Autodesk Inventor part; units mm, degrees
ref_plane "YZ Plane" through (0, 0, 0) normal (1, 0, 0) x (0, 1, 0)
ref_plane "XZ Plane" through (0, 0, 0) normal (0, 1, 0) x (-1, 0, 0)
ref_plane "XY Plane" through (0, 0, 0) normal (0, 0, 1) x (1, 0, 0)
sketch "Boceto1" plane through (0, 0, 0) normal (0, 1, 0) x (-1, 0, 0)
  circle A0 centre (0, 0) radius 1.55
  line L0 (0, 0) -> (0, -1.55)
  line L1 (0, -19.075) -> (0, -14.075)
  line L2 (0, 19.075) -> (0, 16.575)
  arc A1 (2.4369, 17.1331) -> (-2.4369, 17.1331) centre (0, 16.575) ccw
  line L3 (0, -19.075) -> (0, -16.575)
  arc A2 (-2.4369, -17.1331) -> (2.4369, -17.1331) centre (0, -16.575) ccw
  line L4 (-2.4369, 17.1331) -> (-6.0436, 1.384)
  line L5 (2.4369, 17.1331) -> (6.0436, 1.384)
  line L6 (2.4369, -17.1331) -> (6.0436, -1.384)
  line L7 (-2.4369, -17.1331) -> (-6.0436, -1.384)
  arc A3 (-6.0436, 1.384) -> (-6.0436, -1.384) centre (0, 0) ccw
  arc A4 (6.0436, -1.384) -> (6.0436, 1.384) centre (0, 0) ccw
  dimension "d0" = 3.1
  dimension "d2" = 19.075
  dimension "d3" = 38.15
  dimension "d4" = 2.5
  dimension "d5" = 2.5
extrude "Extrusión1" add sketch "Boceto1" along normal blind 2.3
sketch "Boceto2" plane through (0, 2.3, 0) normal (0, 1, 0) x (1, 0, 0)
  circle A0 centre (0, 0) radius 1.55
  circle A1 centre (0, 0) radius 4.35
  circle A2 centre (0, 0) radius 2.7
  dimension "d8" = 8.7
  dimension "d9" = 5.4
extrude "Extrusión2" add sketch "Boceto2" along normal blind 3.3 contours A1
sketch "Boceto3" plane through (0, 0, 0) normal (0, -1, 0) x (1, 0, 0)
  circle A0 centre (0, 0) radius 1.55
  line L0 (0, -1.55) -> (0, 1.55)
properties part number "Brazo"
CAD build for the part. Positions are in the model's coordinates, mm. Coordinates: 2 decimals unless noted, no trailing zeros. Write each loop counter-clockwise with the first axis right and the second up, starting at its lowest first coordinate (ties: lowest second). Pieces come first, ordered by that corner, then holes.
(1) Flat gauge pins, fed straight in: pin 1 (6 mm diameter, centred on x = 0, z = 2.5, fed in from +Y); pin 2 (2.5 mm diameter, centred on x = 0, z = -0.5, fed in from +Y); pin 3 (2 mm diameter, centred on x = 3, y = 3.5, fed in from +Z). Where does each tip first touch, or does it go through?
(2) Cut at B-B, the plane z = 0. List the corners of the cut face in (x, y), and give its area (3 significant figures).
(3) Two-plate mould, pull along X, no slides. Class faces 1 (the face through (0, 2.3, -2)), 2 (the face through (-0.943, 3.927, -4.247)), 3 (the face through (-0.585, 3.927, -2.636)), 4 (the face through (0, 2.3, 5)): +X half, -X half, draft (parallel to the pull), parting line (faces both ways), or undercut.
(4) Cut at C-C, the plane y = 5.2. List the corners of the cut face in (x, z).
(5) Cut at A-A, the plane x = 0. List the corners of the cut face in (y, z) (3 decimals).
(6) Cut at D-D, the plane x = 4. List the corners of the cut face in (y, z).
(7) Drill centre lines: probe 1 along X at (y, z) = (4.6, 0); probe 2 along Z at (x, y) = (0, 1.3) (3 decimals). Where is each one in solid material? Low to high.
Geometry says:
1. pin 1: stops at y = 5.6
1. pin 2: stops at y = 2.3
1. pin 3: stops at z = 3.86
2. outline: (-6.2, 0) - (-1.55, 0) - (-1.55, 2.3) - (-2.7, 2.3) - (-2.7, 5.6) - (-4.35, 5.6) - (-4.35, 2.3) - (-6.2, 2.3) - close; (1.55, 0) - (6.2, 0) - (6.2, 2.3) - (4.35, 2.3) - (4.35, 5.6) - (2.7, 5.6) - (2.7, 2.3) - (1.55, 2.3) - close
2. area: 32.3 mm2
3. face 1: undercut
3. face 2: parting line
3. face 3: undercut
3. face 4: draft
4. outline: circle Ø8.7 at (0, 0); hole circle Ø5.4 at (0, 0)
5. outline: (0, -19.075) - (2.3, -19.075) - (2.3, -4.35) - (5.6, -4.35) - (5.6, -2.7) - (2.3, -2.7) - (2.3, -1.55) - (0, -1.55) - close; (0, 1.55) - (2.3, 1.55) - (2.3, 2.7) - (5.6, 2.7) - (5.6, 4.35) - (2.3, 4.35) - (2.3, 19.075) - (0, 19.075) - close
6. outline: (0, -10.31) - (2.3, -10.31) - (2.3, -1.71) - (5.6, -1.71) - (5.6, 1.71) - (2.3, 1.71) - (2.3, 10.31) - (0, 10.31) - close
7. probe 1: x = -4.35 to -2.7, 2.7 to 4.35
7. probe 2: z = -19.075 to -1.55, 1.55 to 19.075
